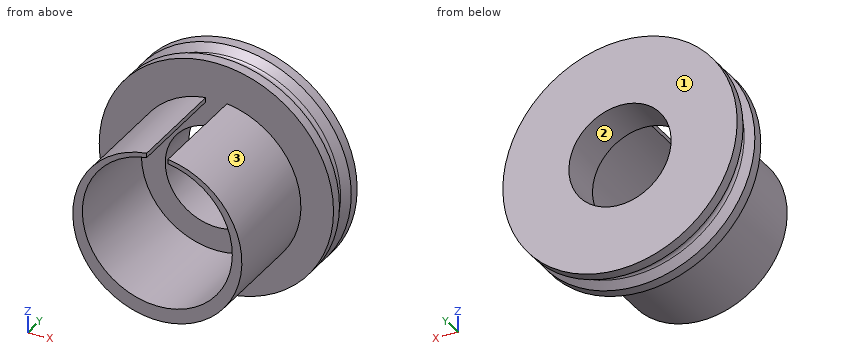
```python
from build123d import *

# Parameters (mm, degrees)
SKETCH1_R           = 12.6
SKETCH1_R_2         = 11.176
BOSS_EXTRUDE1_DEPTH = 15.875
SKETCH2_R           = 17.4625
SKETCH2_R_2         = 7.62
BOSS_EXTRUDE2_DEPTH = 6.35
SKETCH4_W           = 3.175
SKETCH4_H           = 15.94800196
CUT_EXTRUDE1_DEPTH  = 15.875


with BuildPart() as part:
    # Sketch1 → Boss-Extrude1 (new body)
    with BuildSketch(Plane(origin=(0, 0, 0), x_dir=(1, 0, 0), z_dir=(0, 1, 0))):
        with Locations(Location((0, 0.762, 0), (0, 0, 270))):
            Circle(SKETCH1_R)
        with Locations(Location((0, 0, 0), (0, 0, 270))):
            Circle(SKETCH1_R_2, mode=Mode.SUBTRACT)
    extrude(amount=BOSS_EXTRUDE1_DEPTH)

    # Sketch2 → Boss-Extrude2 (add)
    with BuildSketch(Plane(origin=(0, 15.875, 0), x_dir=(1, 0, 0), z_dir=(0, 1, 0))):
        with Locations(Location((0, 0, 0), (0, 0, 270))):
            Circle(SKETCH2_R)
        with Locations(Location((0, 0, 0), (0, 0, 270))):
            Circle(SKETCH2_R_2, mode=Mode.SUBTRACT)
    extrude(amount=BOSS_EXTRUDE2_DEPTH)

    # Sketch3 → Cut-Revolve1 (revolve, cut)
    with BuildSketch(Plane.XY, mode=Mode.PRIVATE) as cut_revolve1_sk:
        with BuildLine():
            Line((-17.4625, 20.6375), (-16.436266008, 19.611266008))
            ThreePointArc((-16.436266008, 19.611266008), (-16.203782015, 19.05), (-16.436266008, 18.488733992))
            Line((-16.436266008, 18.488733992), (-17.4625, 17.4625))
            Line((-17.4625, 17.4625), (-17.4625, 20.6375))
        make_face()
    revolve(cut_revolve1_sk.sketch.rotate(Axis((0, 22.225, 0), (0, -1, 0)), 270), axis=Axis((0, 22.225, 0), (0, -1, 0)), mode=Mode.SUBTRACT)

    # Sketch4 → Cut-Extrude1 (cut)
    with BuildSketch(Plane.XZ):
        with Locations((0, 11.838)):
            Rectangle(SKETCH4_W, SKETCH4_H)
    extrude(amount=-CUT_EXTRUDE1_DEPTH, mode=Mode.SUBTRACT)


solid = part.part
```
Check sheet for the modelled part. Datum: model origin and axes. Units: mm. Face numbers are marked on the shaded views. Round coordinates to 2 decimals unless told otherwise and drop trailing zeros. Order: outer loops, then holes, each group sorted by start corner. A loop starts at its lowest first (then second) coordinate and runs counter-clockwise, first axis right, second up.
1) Go/stop test with flat-tipped pins: pin 1 Ø3 at (y, z) = (14, -11.5) entering from +X; pin 2 Ø3 at (y, z) = (16, 8.5) entering from +X; pin 3 Ø8 at (x, y) = (7.5, 2) entering from -Z; pin 4 Ø13.5 at (x, z) = (0, 0) entering from +Y. Record where each tip stops, or that it passes through.
2) Scan lines: line 1 (Y direction, x = -9.5, z = -10) (3 decimals); line 2 (Z direction, x = 9.5, y = 8.25); line 3 (X direction, y = 19.5, z = 0). Record each from-to range of solid material in increasing order.
3) Mould release check, pull along Z, two halves, no side actions. Record for the marked faces 1, 2 and 3: +Z half, -Z half, draft (parallel to the pull), parting line (faces both ways), or undercut.
4) Section check D-D (y = 11.5). Record the boundary of the cut face in (x, z).
5) Section check C-C (y = 16.75). Record the boundary of the cut face in (x, z) (1 decimal).
Result:
1. pin 1: stops at x = 8.57
1. pin 2: stops at x = 16
1. pin 3: stops at z = -12.87
1. pin 4: passes through
2. line 1: y = 15.875 to 22.225
2. line 2: z = -9.04 to -5.89, 5.89 to 7.52
2. line 3: x = -16.34 to -7.62, 7.62 to 16.34
3. face 1: draft
3. face 2: undercut
3. face 3: parting line
4. outline: (-1.59, 11.06) - (-1.59, 11.74) arc R12.6 ccw (long way) to (1.59, 11.74) - (1.59, 11.06) arc R11.18 cw (long way) to start
5. outline: circle Ø34.9 at (0, 0); hole circle Ø15.2 at (0, 0)
